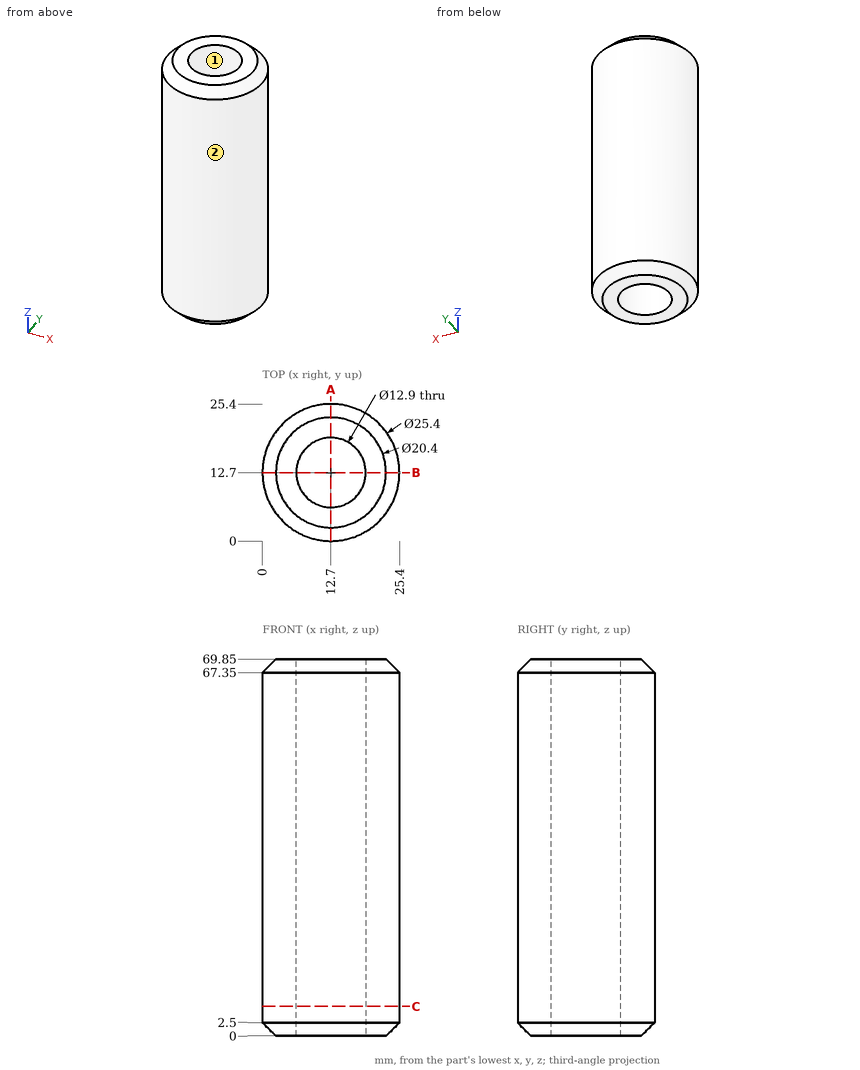
The figure shows three views and two pictorial views of one solid part (mm, origin at its lowest corner). Answer the questions. Round coordinates to 2 decimals unless told otherwise and drop trailing zeros. Write each loop counter-clockwise with the first axis right and the second up, starting at its lowest first coordinate (ties: lowest second). Pieces come first, ordered by that corner, then holes. Notation, with made-up numbers: M 45,-34 L 89,-34 A19 cw 89,-28 Z; hole C 83,6.25 d6. An arc over 180 degrees is marked long. Use a Markdown table: item, result.
1) The part is cut by section C-C on z = 5.5. Give the vertices of the cut face in (x, y).
Taken from the geometry:
| item | result |
|---|---|
| outline | C 12.7,12.7 d25.4; hole C 12.7,12.7 d12.9 |
2) Determine the mould class of the marked faces 1 and 2 for opening direction Y: pulls with the +Y half, pulls with the -Y half, needs draft (parallel to the pull), parting line crosses it, or undercut.
Taken from the geometry:
| item | result |
|---|---|
| face 1 | undercut |
| face 2 | parting line crosses it |
3) Flat-ended cylindrical pins translate along their axes: pin 1 (3 mm diameter, centred on y = 4.5, z = 39.5, fed in from -X); pin 2 (4 mm diameter, centred on y = 19.5, z = 36, fed in from +X); pin 3 (1 mm diameter, centred on y = 16.5, z = 56.5, fed in from -X). Find the tip coordinate at first contact, or state that the pin passes through.
Taken from the geometry:
| item | result |
|---|---|
| pin 1 | stops at x = 1.91 |
| pin 2 | stops at x = 24.46 |
| pin 3 | stops at x = 0.44 |
4) The part is cut by section A-A on x = 12.7. Give the vertices of the cut face in (y, z).
Taken from the geometry:
| item | result |
|---|---|
| outline | M 0,2.5 L 2.5,0 L 6.25,0 L 6.25,69.85 L 2.5,69.85 L 0,67.35 Z; M 19.15,0 L 22.9,0 L 25.4,2.5 L 25.4,67.35 L 22.9,69.85 L 19.15,69.85 Z |
5) Consider line 1 (Y direction, x = 12.7, z = 16); line 2 (Y direction, x = 11.25, z = 65); line 3 (X direction, y = 9.5, z = 67.5). Determine where each line is inside the solid, lowest interval first. Write a range as [from, to].
Taken from the geometry:
| item | result |
|---|---|
| line 1 | y = [0, 6.25], [19.15, 25.4] |
| line 2 | y = [0.08, 6.42], [18.98, 25.32] |
| line 3 | x = [0.56, 7.1], [18.3, 24.84] |
